Work out the finished part from the listing and answer in its coordinate system (mm). A direction names the side the tool comes from. Coordinates: 2 decimals unless noted, no trailing zeros. Order: outer loops, then holes, each group sorted by start corner. A loop starts at its lowest first (then second) coordinate and runs counter-clockwise, first axis right, second up. Notation, with made-up numbers: M -36.5,12 L 2.5,12 A14 cw 2.5,37 Z; hole C 20.25,-15.75 d3. An arc over 180 degrees is marked long. Write item = value, one per line. Start each with the question number.
Q1. Find section B-B on y = -39.5. Give the vertices of the cut face in (x, z).
Q2. Find section C-C on y = 14.5. Give the vertices of the cut face in (x, z).
Q3. Determine the mould class of faces 1 (the flat face through (48, 0, 30)), 2 (the flat face through (-1, 34, 19)), 3 (the flat face through (-1, 35, 98)) for opening direction Y: released by +Y, released by -Y, zero draft, split by the parting line, or undercut.
Q4. A tool of negligible diameter and unlimited length cuts with its end or side. For faces 4 (the flat face through (-11.8, -50, 103.5)), 5 (the flat face through (-48, 0, 30)), 6 (the cylindrical face through (-2.343, 43.86, 17.847)), 7 (the flat face through (-1, -34, 19)), 8 (the flat face through (-1, -35, 98)), from which of +Z, -Z, +X, -X, +Y, -Y can it reach the whole face along a straight path? Write none if from no direction.
Q5. Straight lines are drawn through the part: line 1 along Z through (x, y) = (0, -42); line 2 along Y through (x, z) = (12, 148.5); line 3 along Z through (x, y) = (11, -42) (3 decimals). For each, find the intervals that lie inside material, in ascending order.
Q6. Each of these flat-tipped pins is pushed along its axis until it touches: P1, Ø12, axis at x = -31.5, z = 34, coming from the -Y side; P2, Ø5, axis at x = 17, z = 143.5, coming from the -Y side; P3, Ø8, axis at y = -41, z = 7.5, coming from the +X side. Where does it stop, or does it pass through?
Q7. Find section A-A on x = 0. Give the vertices of the cut face in (y, z), and give its area (3 significant figures).
Q8. Find section D-D on z = 131. Give the vertices of the cut face in (x, y) (3 decimals).
```python
from build123d import *

# Parameters (mm, degrees)
PAD_DEPTH       = 34
SKETCH001_R     = 18
PAD001_DEPTH    = 20
SKETCH002_W     = 100
SKETCH002_H     = 100
PAD002_DEPTH    = 20
PAD003_DEPTH    = 50
SKETCH004_R     = 20
POCKET_DEPTH    = 100
SKETCH005_W     = 100
SKETCH005_H     = 101
POCKET001_DEPTH = 35
SKETCH006_W     = 100
SKETCH006_H     = 10
POCKET002_DEPTH = 16
SKETCH007_W     = 10
SKETCH007_H     = 68
POCKET003_DEPTH = 2


with BuildPart() as part:
    # Sketch → Pad (new body, symmetric)
    with BuildSketch(Plane.XZ):
        with BuildLine():
            ThreePointArc((-48, 0), (0, -48), (48, 0))
            Line((48, 50), (48, 0))
            Line((-48, 50), (48, 50))
            Line((-48, 0), (-48, 50))
        make_face()
    extrude(amount=PAD_DEPTH, both=True)

    # Sketch001 (on Face6 of Pad) → Pad001 (join)
    with BuildSketch(Plane.XZ.offset(34)):
        Circle(SKETCH001_R)
    pad001 = extrude(amount=PAD001_DEPTH)

    # Mirrored: Pad001 across XZ
    add(pad001.mirror(Plane.XZ))

    # Sketch002 (on Face6 of Mirrored) → Pad002 (join)
    with BuildSketch(Plane(origin=(0, 0, 50), x_dir=(-1, 0, 0), z_dir=(0, 0, 1))):
        Rectangle(SKETCH002_W, SKETCH002_H)
    extrude(amount=PAD002_DEPTH)

    # Sketch003 → Pad003 (join, symmetric)
    with BuildSketch(Plane.XZ):
        with BuildLine():
            ThreePointArc((50, 120), (0, 170), (-50, 120))
            Line((-50, 70), (-50, 120))
            Line((50, 70), (-50, 70))
            Line((50, 120), (50, 70))
        make_face()
    extrude(amount=PAD003_DEPTH, both=True)

    # Sketch004 (on Face5 of Pad003) → Pocket (cut)
    with BuildSketch(Plane.XZ.offset(50)):
        with Locations((0, 120)):
            Circle(SKETCH004_R)
    extrude(amount=-POCKET_DEPTH, mode=Mode.SUBTRACT)

    # Sketch005 → Pocket001 (cut, symmetric)
    with BuildSketch(Plane.XZ):
        with Locations((0, 120.5)):
            Rectangle(SKETCH005_W, SKETCH005_H)
    extrude(amount=POCKET001_DEPTH, both=True, mode=Mode.SUBTRACT)

    # Sketch006 (on Face1 of Pocket001) → Pocket002 (cut)
    with BuildSketch(Plane.XZ.offset(50)):
        with Locations((0, 55)):
            Rectangle(SKETCH006_W, SKETCH006_H)
    pocket002 = extrude(amount=-POCKET002_DEPTH, mode=Mode.SUBTRACT)

    # Mirrored001: Pocket002 across XZ
    add(pocket002.mirror(Plane.XZ), mode=Mode.SUBTRACT)

    # Sketch007 (on Face3 of Mirrored001) → Pocket003 (cut)
    with BuildSketch(Plane(origin=(-50, 0, 0), x_dir=(0, 0, -1), z_dir=(-1, 0, 0))):
        with Locations((-55, 0)):
            Rectangle(SKETCH007_W, SKETCH007_H)
    pocket003 = extrude(amount=-POCKET003_DEPTH, mode=Mode.SUBTRACT)

    # Mirrored002: Pocket003 across YZ
    add(pocket003.mirror(Plane.YZ), mode=Mode.SUBTRACT)


solid = part.part
```
Findings below:
q1.outline = M -50,60 L 50,60 L 50,120 A50 ccw -50,120 Z; C 0,0 d36; hole C 0,120 d40
q2.outline = M -50,60 L -48,60 L -48,0 A48 ccw 48,0 L 48,60 L 50,60 L 50,70 L -50,70 Z
q3.face_1 = zero draft
q3.face_2 = released by +Y
q3.face_3 = undercut
q4.face_4 = +Z, +X, -X, -Y
q4.face_5 = -Z, -X, +Y, -Y
q4.face_6 = +Y
q4.face_7 = -Y
q4.face_8 = +Z, +X, -X
q5.line_1 = -18 to 18, 60 to 100, 140 to 170
q5.line_2 = -50 to -35, 35 to 50
q5.line_3 = -14.248 to 14.248, 60 to 103.297, 136.703 to 168.775
q6.P1 = -34
q6.P2 = -50
q6.P3 = 17.66
q7.outline = M -54,-18 L -34,-18 L -34,-48 L 34,-48 L 34,-18 L 54,-18 L 54,18 L 34,18 L 34,60 L 50,60 L 50,100 L 35,100 L 35,70 L -35,70 L -35,100 L -50,100 L -50,60 L -34,60 L -34,18 L -54,18 Z; M -50,140 L -35,140 L -35,170 L -50,170 Z; M 35,140 L 50,140 L 50,170 L 35,170 Z
q7.area = 11,600 mm^2
q8.outline = M -48.775,-50 L -16.703,-50 L -16.703,-35 L -48.775,-35 Z; M -48.775,35 L -16.703,35 L -16.703,50 L -48.775,50 Z; M 16.703,-50 L 48.775,-50 L 48.775,-35 L 16.703,-35 Z; M 16.703,35 L 48.775,35 L 48.775,50 L 16.703,50 Z
